Read the model definition and answer for the solid it produces. Units are mm, in the model's axes. A direction names the side the tool comes from. Give positions to 0.01 mm unless a question says otherwise; leave off trailing zeros. Order: outer loops, then holes, each group sorted by start corner. A loop starts at its lowest first (then second) coordinate and runs counter-clockwise, first axis right, second up. Notation, with made-up numbers: (75, -21.5) - (130, -21.5) arc R32 ccw to (130, 15.5) - close; hole circle Ø8 at (-37.5, 35.25). An arc over 180 degrees is marked (long way). Return JSON: item names as keys, results as strings.
```python
from build123d import *

# Parameters (mm, degrees)
SKETCH1_W           = 20
SKETCH1_H           = 3.175
BOSS_EXTRUDE1_DEPTH = 3.175


with BuildPart() as part:
    # Sketch1 → Boss-Extrude1 (new body)
    with BuildSketch(Plane(origin=(0, 0, 0), x_dir=(0, 0, -1), z_dir=(1, 0, 0))):
        with Locations((0, 14.5875)):
            Rectangle(SKETCH1_W, SKETCH1_H)
        Polygon((-24.5, 13), (-24.5, -13), (-10, -13), (10, -13), (24.5, -13), (24.5, 13), (10, 13), (-10, 13), align=None)
        with Locations((0, -14.5875)):
            Rectangle(SKETCH1_W, SKETCH1_H)
    extrude(amount=BOSS_EXTRUDE1_DEPTH)


solid = part.part
```
Q1. A cutting plane is placed at B-B (z = -17). Write down the section's boundary in (x, y) (3 decimals), and give its area (4 significant figures).
Values:
{"outline": "(0, -13) - (3.175, -13) - (3.175, 13) - (0, 13) - close", "area": "82.55 mm²"}
Q2. Given pin 1 (1.6 mm diameter, centred on x = 2, z = -15.5, fed in from +Y); pin 2 (1.6 mm diameter, centred on x = 1, z = 14.5, fed in from -Y); pin 3 (1 mm diameter, centred on x = 2, y = 15, fed in from +Z), each flat-ended and moving along its own axis, determine where each tip first touches the part or whether it passes through.
Values:
{"pin 1": "stops at y = 13", "pin 2": "stops at y = -13", "pin 3": "stops at z = 10"}
Q3. A cutting plane is placed at C-C (y = 13.5). Write down the section's boundary in (x, z) (3 decimals).
Values:
{"outline": "(0, -10) - (3.175, -10) - (3.175, 10) - (0, 10) - close"}
Q4. Consider L1, parallel to Y at x = 1.25, z = -12.5; L2, parallel to Z at x = 1.7, y = -14.5. Determine where each line is inside the solid, lowest interval first.
Values:
{"L1": "y = -13 to 13", "L2": "z = -10 to 10"}
Q5. A cutting plane is placed at A-A (x = 1.55). Write down the section's boundary in (y, z) (3 decimals), and give its area (3 significant figures).
Values:
{"outline": "(-16.175, -10) - (-13, -10) - (-13, -24.5) - (13, -24.5) - (13, -10) - (16.175, -10) - (16.175, 10) - (13, 10) - (13, 24.5) - (-13, 24.5) - (-13, 10) - (-16.175, 10) - close", "area": "1,400 mm²"}
Q6. For faces 1 (the flat face through (2, -13, -17)), 2 (the flat face through (2, -13, 17)), 3 (the flat face through (2, 15, 10)), determine the directions among +Z, -Z, +X, -X, +Y, -Y from which every point of the face is accessible in a straight line to the end or side of a thin tool.
Values:
{"face 1": "-Z, +X, -X, -Y", "face 2": "+Z, +X, -X, -Y", "face 3": "+Z, +X, -X, +Y"}
